The listing builds one solid part. Answer for the finished solid, in the listing's coordinates (mm). Give positions to 0.01 mm unless a question says otherwise; leave off trailing zeros. Loops run counter-clockwise (first coordinate to the right, second up) from the corner with the lowest first, then second, coordinate; pieces in that order, holes last. Notation, with made-up numbers: (35, 55.5) - (66, 55.5) arc R18 ccw to (66, 76.5) - close; hole circle Ø1 at (-36, 57). An arc over 180 degrees is marked (long way). Write item = value, one per line. Start each with the question number.
1) Consider probe 1 along X at (y, z) = (3, -180.5); probe 2 along Z at (x, y) = (225, 9.5); probe 3 along Z at (x, y) = (201.5, 1.25). Determine where each line is inside the solid, lowest interval first.
2) The part is cut by section A-A on x = 20. Write down the section's boundary in (y, z), plus the area to 3 significant figures.
3) Flat-ended cylindrical pins translate along their axes: P1, Ø3, axis at y = 7, z = 186.5, coming from the -X side; P2, Ø3, axis at x = 246.5, y = 5, coming from the -Z side; P3, Ø5, axis at y = 3, z = 180.5, coming from the +X side. Find the tip coordinate at first contact, or state that the pin passes through.
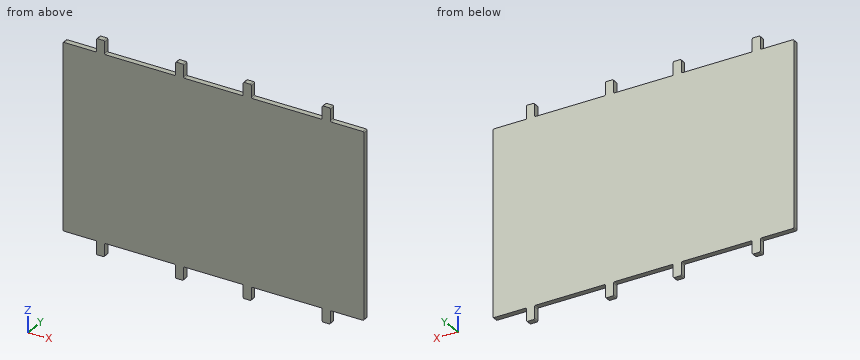
from build123d import *

# Parameters (mm, degrees)
SKETCH1_W               = 560
SKETCH1_H               = 344
BOSS_EXTRUDE1_DEPTH     = 10
SKETCH2_W               = 15
SKETCH2_H               = 25
BOSS_EXTRUDE2_DEPTH     = 10
MIRROR5_COPY_1_SKETCH_W = 15
MIRROR5_COPY_1_SKETCH_H = 25
MIRROR5_COPY_1_DEPTH    = 10
FILLET3_R               = 2


with BuildPart() as part:
    # Sketch1 → Boss-Extrude1 (new body)
    with BuildSketch(Plane(origin=(0, 0, 0), x_dir=(1, 0, 0), z_dir=(0, 1, 0))):
        Rectangle(SKETCH1_W, SKETCH1_H)
    extrude(amount=BOSS_EXTRUDE1_DEPTH)

    # Sketch2 → Boss-Extrude2 (add)
    with BuildSketch(Plane(origin=(0, 10, 0), x_dir=(1, 0, 0), z_dir=(0, 1, 0))):
        with Locations((-63, -184.5)):
            Rectangle(SKETCH2_W, SKETCH2_H)
        with Locations((-210, -184.5)):
            Rectangle(SKETCH2_W, SKETCH2_H)
    boss_extrude2 = extrude(amount=-BOSS_EXTRUDE2_DEPTH)

    # Mirror4: Boss-Extrude2 across plane
    add(boss_extrude2.mirror(Plane(origin=(0, 0, 0), x_dir=(0, 0, 1), z_dir=(1, 0, 0))))

    # Mirror5: Boss-Extrude2 across plane
    add(boss_extrude2.mirror(Plane.XY))

    # Mirror5 copy 1 sketch → Mirror5 copy 1 (add)
    with BuildSketch(Plane(origin=(0, 10, 0), x_dir=(-1, 0, 0), z_dir=(0, 1, 0))):
        with Locations((-63, -184.5)):
            Rectangle(MIRROR5_COPY_1_SKETCH_W, MIRROR5_COPY_1_SKETCH_H)
        with Locations((-210, -184.5)):
            Rectangle(MIRROR5_COPY_1_SKETCH_W, MIRROR5_COPY_1_SKETCH_H)
    extrude(amount=-MIRROR5_COPY_1_DEPTH)

    # Fillet3
    fillet3_edges = [part.edges().sort_by_distance(p)[0] for p in [
        (-70.5, 5, 197),
        (-70.5, 5, 172),
        (-55.5, 5, 172),
        (-55.5, 5, 197),
        (-202.5, 5, 172),
        (-202.5, 5, 197),
        (-217.5, 5, 197),
        (-217.5, 5, 172),
        (55.5, 5, 172),
        (55.5, 5, 197),
        (70.5, 5, 197),
        (70.5, 5, 172),
        (217.5, 5, 197),
        (217.5, 5, 172),
        (202.5, 5, 172),
        (202.5, 5, 197),
        (70.5, 5, -197),
        (70.5, 5, -172),
        (55.5, 5, -172),
        (55.5, 5, -197),
        (202.5, 5, -172),
        (202.5, 5, -197),
        (217.5, 5, -197),
        (217.5, 5, -172),
        (-280, 5, -172),
        (280, 5, -172),
        (280, 5, 172),
        (-280, 5, 172),
        (-55.5, 5, -172),
        (-55.5, 5, -197),
        (-70.5, 5, -197),
        (-70.5, 5, -172),
        (-217.5, 5, -197),
        (-217.5, 5, -172),
        (-202.5, 5, -172),
        (-202.5, 5, -197),
    ]]
    fillet(fillet3_edges, radius=FILLET3_R)


solid = part.part
Answer below:
q1.probe_1 = -217.5 to -202.5, -70.5 to -55.5, 55.5 to 70.5, 202.5 to 217.5
q1.probe_2 = -172 to 172
q1.probe_3 = -172.27 to 172.27
q2.outline = (0, -172) - (10, -172) - (10, 172) - (0, 172) - close
q2.area = 3,440 mm2
q3.P1 = -217.5
q3.P2 = -172
q3.P3 = 217.5
